Source: CAD feature listing. Evaluate the final solid. Frame: model axes, mm. A direction names the side the tool comes from. Give positions to 0.01 mm unless a question says otherwise; leave off trailing zeros. Order: outer loops, then holes, each group sorted by start corner. A loop starts at its lowest first (then second) coordinate and runs counter-clockwise, first axis right, second up. Notation, with made-up numbers: (58.5, 0.5) - (82.5, 0.5) arc R25 cw to (82.5, 27.5) - close; hole circle Ø2 at (23.25, 74.25). An arc over 180 degrees is marked (long way). Use CSV: the item, a comma, the result in double quotes.
```python
from build123d import *

# Parameters (mm, degrees)
F0_W     = 55
F0_H     = 43
F1_DEPTH = 2
F2_W     = 43
F2_H     = 18
F2_W_2   = 12
F2_H_2   = 2.5
F2_W_3   = 18
F2_H_3   = 16
F3_DEPTH = 9
F5_DEPTH = 6
F6_W     = 9
F6_H     = 6
F7_DEPTH = 1.5


with BuildPart() as f1:
    # F0 (on Top) → F1 (new body)
    with BuildSketch(Plane.XY):
        Rectangle(F0_W, F0_H)
    extrude(amount=F1_DEPTH)

    # F2 (on face) → F3 (join)
    with BuildSketch(Plane.XY.offset(2)):
        with Locations((-3, 6.5)):
            Rectangle(F2_W, F2_H)
        with Locations((1.5, -6.75)):
            Rectangle(F2_W_2, F2_H_2)
        with Locations((17.5, -12.5)):
            Rectangle(F2_W_3, F2_H_3)
        with BuildLine():
            ThreePointArc((-15.5, -15.5), (-17.5, -13.5), (-19.5, -15.5))
            Line((-19.5, -15.5), (-15.5, -15.5))
        make_face()
    extrude(amount=F3_DEPTH)

    # F4 (on face) → F5 (cut)
    with BuildSketch(Plane.XY.offset(11)):
        Polygon((-22.5, 13.5), (-22.5, 15.5), (-24.5, 15.5), (-24.5, 11), (-16.5, 11), (-16.5, 2), (-24.5, 2), (-24.5, -2.5), (-22.5, -2.5), (-22.5, -0.5), (16.5, -0.5), (16.5, -2.5), (18.5, -2.5), (18.5, 15.5), (16.5, 15.5), (16.5, 13.5), align=None)
        Polygon((10.5, -4.5), (8.5, -4.5), (8.5, -20.5), (10.5, -20.5), (10.5, -18.5), (24.5, -18.5), (24.5, -20.5), (26.5, -20.5), (26.5, -4.5), (24.5, -4.5), (24.5, -6.5), (10.5, -6.5), align=None)
    extrude(amount=-F5_DEPTH, mode=Mode.SUBTRACT)

    # F6 (on face) → F7 (join)
    with BuildSketch(Plane(origin=(-24.5, 0, 0), x_dir=(0, -1, 0), z_dir=(-1, 0, 0))):
        with Locations((-6.5, 8)):
            Rectangle(F6_W, F6_H)
    extrude(amount=F7_DEPTH)


solid = f1.part
```
Item 1: First-contact query: pin 1 (3 mm diameter, centred on x = -3.5, z = 8, fed in from -Y); pin 2 (4 mm diameter, centred on x = -7, z = 7.5, fed in from +Y); pin 3 (1.5 mm diameter, centred on x = 17.5, z = 4.5, fed in from -Y); pin 4 (4 mm diameter, centred on x = -5.5, y = -16, fed in from -Z). Flat tips, straight axial feed; report the tip coordinate or a pass-through.
Filled in:
pin 1,"stops at y = -8"
pin 2,"stops at y = 15.5"
pin 3,"stops at y = -20.5"
pin 4,"stops at z = 0"
Item 2: Section B-B on x = -17.5. Return the cut outline in (y, z).
Filled in:
outline,"(-21.5, 0) - (21.5, 0) - (21.5, 2) - (15.5, 2) - (15.5, 11) - (13.5, 11) - (13.5, 5) - (11, 5) - (11, 11) - (2, 11) - (2, 5) - (-0.5, 5) - (-0.5, 11) - (-2.5, 11) - (-2.5, 2) - (-13.5, 2) - (-13.5, 11) - (-15.5, 11) - (-15.5, 2) - (-21.5, 2) - close"
Item 3: Material intervals for line 1 (Y direction, x = 13, z = 6.75); line 2 (Y direction, x = -21.5, z = 6.75); line 3 (Z direction, x = -25, y = 10.5), sorted ascending. Write a range as from..to.
Filled in:
line 1,"y = -20.5..-18.5, -6.5..-4.5, -2.5..-0.5, 13.5..15.5"
line 2,"y = -2.5..-0.5, 2..11, 13.5..15.5"
line 3,"z = 0..2, 5..11"
Item 4: Section C-C on z = 3.25. Return the cut outline in (x, y), then the cut area to 3 significant figures.
Filled in:
outline,"(-24.5, -2.5) - (18.5, -2.5) - (18.5, 15.5) - (-24.5, 15.5) - close; (-19.5, -15.5) - (-15.5, -15.5) arc R2 ccw to start; (-4.5, -8) - (7.5, -8) - (7.5, -5.5) - (-4.5, -5.5) - close; (8.5, -20.5) - (26.5, -20.5) - (26.5, -4.5) - (8.5, -4.5) - close"
area,"1,100 mm2"
Item 5: Mould query, pull axis Y, two halves, no side actions, for faces 5 (the flat face through (17, -20.5, 6)), 6 (the flat face through (27.5, 0, 1)), 7 (the cylindrical face through (-17.5, -13.5, 6.4)). Classes: released by +Y, released by -Y, zero draft, split by the parting line, or undercut.
Filled in:
face 5,"released by -Y"
face 6,"zero draft"
face 7,"undercut"
Item 6: Section A-A on z = 10. Return the cut outline in (x, y), then the cut area to 3 significant figures.
Filled in:
outline,"(-26, 2) - (-16.5, 2) - (-16.5, 11) - (-26, 11) - close; (-22.5, -2.5) - (16.5, -2.5) - (16.5, -0.5) - (-22.5, -0.5) - close; (-22.5, 13.5) - (16.5, 13.5) - (16.5, 15.5) - (-22.5, 15.5) - close; (-19.5, -15.5) - (-15.5, -15.5) arc R2 ccw to start; (-4.5, -8) - (7.5, -8) - (7.5, -5.5) - (-4.5, -5.5) - close; (10.5, -20.5) - (24.5, -20.5) - (24.5, -18.5) - (10.5, -18.5) - close; (10.5, -6.5) - (24.5, -6.5) - (24.5, -4.5) - (10.5, -4.5) - close"
area,"334 mm2"
Item 7: Set-up query: faces 1 (the flat face through (26.5, -13, 3)), 2 (the flat face through (16.5, 15, 8)), 3 (the flat face through (-16.5, 7, 8)), 4 (the flat face through (10.5, -6, 8)). Return all of +Z, -Z, +X, -X, +Y, -Y with unobstructed straight access to the full face (end or side cutting, diameter ignored); none if empty.
Filled in:
face 1,"+Z, +X, +Y, -Y"
face 2,"+Z, +X, +Y"
face 3,"+Z, +X"
face 4,"+Z, -Y"
